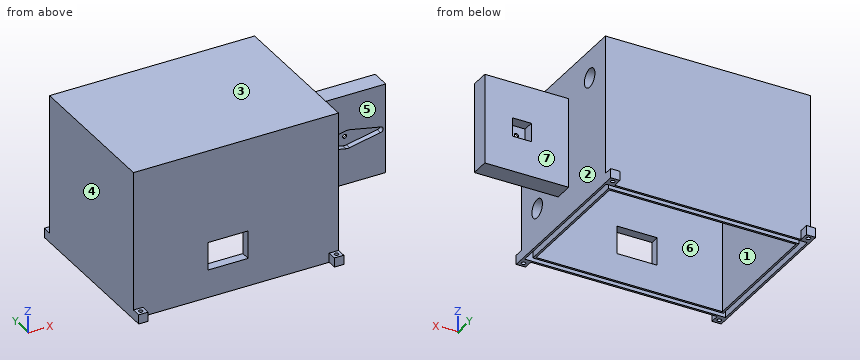
```python
from build123d import *

# Parameters (mm, degrees)
SKETCH_1_W           = 155
SKETCH_1_H           = 80
EXTRUDE_1_DEPTH      = 80
SKETCH_6_W           = 45
SKETCH_6_H           = 80
CUT_EXTRUDE_1_DEPTH  = 35
SKETCH_5_W           = 45
SKETCH_5_H           = 80
CUT_EXTRUDE_2_DEPTH  = 35
SKETCH_7_W           = 100
SKETCH_7_H           = 70
CUT_EXTRUDE_3_DEPTH  = 75
SKETCH_8_W           = 107.8
SKETCH_8_H           = 77.8
SKETCH_8_W_2         = 102.2
SKETCH_8_H_2         = 72.2
CUT_EXTRUDE_4_DEPTH  = 10
SKETCH_9_R           = 5
CUT_EXTRUDE_5_DEPTH  = 10
SKETCH_10_W          = 21.5
SKETCH_10_H          = 15
CUT_EXTRUDE_6_DEPTH  = 10
SKETCH_12_W          = 15.816906699
SKETCH_12_H          = 10
CUT_EXTRUDE_7_DEPTH  = 45
CUT_EXTRUDE_8_DEPTH  = 3
SKETCH_15_W          = 10
SKETCH_15_H          = 10
CUT_EXTRUDE_9_DEPTH  = 6
SKETCH_17_R          = 1.095275866
CUT_EXTRUDE_11_DEPTH = 7
SKETCH_18_W          = 5
SKETCH_18_H          = 5
SKETCH_18_R          = 1.1
EXTRUDE_2_DEPTH      = 5


with BuildPart() as part:
    # 草圖1 → 填料-伸長1 (new body)
    with BuildSketch(Plane.XY):
        with Locations((1.991097826, 5.58988764)):
            Rectangle(SKETCH_1_W, SKETCH_1_H)
    extrude(amount=EXTRUDE_1_DEPTH)

    # 草圖6 → 除料-伸長1 (cut)
    with BuildSketch(Plane(origin=(0, 45.58988764, 0), x_dir=(1, 0, 0), z_dir=(0, 1, 0))):
        with Locations((56.991097826, -40)):
            Rectangle(SKETCH_6_W, SKETCH_6_H)
    extrude(amount=-CUT_EXTRUDE_1_DEPTH, mode=Mode.SUBTRACT)

    # 草圖5 → 除料-伸長2 (cut)
    with BuildSketch(Plane.XZ.offset(34.41011236)):
        with Locations((56.991097826, 40)):
            Rectangle(SKETCH_5_W, SKETCH_5_H)
    extrude(amount=-CUT_EXTRUDE_2_DEPTH, mode=Mode.SUBTRACT)

    # 草圖7 → 除料-伸長3 (cut)
    with BuildSketch(Plane.XY):
        with Locations((-20.508902174, 5.58988764)):
            Rectangle(SKETCH_7_W, SKETCH_7_H)
    extrude(amount=CUT_EXTRUDE_3_DEPTH, mode=Mode.SUBTRACT)

    # 草圖8 → 除料-伸長4 (cut)
    with BuildSketch(Plane(origin=(0, 0, 0), x_dir=(-1, 0, 0), z_dir=(0, 0, -1))):
        with Locations((20.508902174, 5.58988764)):
            Rectangle(SKETCH_8_W, SKETCH_8_H)
        with Locations((20.508902174, 5.58988764)):
            Rectangle(SKETCH_8_W_2, SKETCH_8_H_2, mode=Mode.SUBTRACT)
    extrude(amount=-CUT_EXTRUDE_4_DEPTH, mode=Mode.SUBTRACT)

    # 草圖9 → 除料-伸長5 (cut)
    with BuildSketch(Plane(origin=(34.491097826, 0, 0), x_dir=(0, 0, -1), z_dir=(1, 0, 0))):
        with Locations((-65, 30.58988764)):
            Circle(SKETCH_9_R)
        with Locations((-20, -19.41011236)):
            Circle(SKETCH_9_R)
    extrude(amount=-CUT_EXTRUDE_5_DEPTH, mode=Mode.SUBTRACT)

    # 草圖10 → 除料-伸長6 (cut)
    with BuildSketch(Plane(origin=(0, -34.41011236, 0), x_dir=(-1, 0, 0), z_dir=(0, -1, 0))):
        with Locations((24.758902174, -22.5)):
            Rectangle(SKETCH_10_W, SKETCH_10_H)
    extrude(amount=-CUT_EXTRUDE_6_DEPTH, mode=Mode.SUBTRACT)

    # 草圖12 → 除料-伸長7 (cut)
    with BuildSketch(Plane(origin=(34.491097826, 0, 0), x_dir=(0, 0, -1), z_dir=(1, 0, 0))):
        with Locations((-72.09154665, 5.58988764)):
            Rectangle(SKETCH_12_W, SKETCH_12_H)
        with Locations((-7.90845335, 5.58988764)):
            Rectangle(SKETCH_12_W, SKETCH_12_H)
    extrude(amount=CUT_EXTRUDE_7_DEPTH, mode=Mode.SUBTRACT)

    # 草圖14 → 除料-伸長8 (cut)
    with BuildSketch(Plane(origin=(0, 0.58988764, 0), x_dir=(-1, 0, 0), z_dir=(0, -1, 0))):
        with BuildLine():
            Line((-58.137150435, -35.10282789), (-41.645964254, -38.5))
            ThreePointArc((-41.645964254, -38.5), (-40.145964254, -40), (-41.645964254, -41.5))
            Line((-41.645964254, -41.5), (-58.137150435, -44.89717211))
            ThreePointArc((-58.137150435, -44.89717211), (-59.145964254, -45), (-60.154778073, -44.89717211))
            Line((-60.154778073, -44.89717211), (-76.645964254, -41.5))
            ThreePointArc((-76.645964254, -41.5), (-78.145964254, -40), (-76.645964254, -38.5))
            Line((-76.645964254, -38.5), (-60.154778073, -35.10282789))
            ThreePointArc((-60.154778073, -35.10282789), (-59.145964254, -35), (-58.137150435, -35.10282789))
        make_face()
    extrude(amount=-CUT_EXTRUDE_8_DEPTH, mode=Mode.SUBTRACT)

    # 草圖15 → 除料-伸長9 (cut)
    with BuildSketch(Plane(origin=(0, 10.58988764, 0), x_dir=(1, 0, 0), z_dir=(0, 1, 0))):
        with Locations((59.491097826, -39.816906699)):
            Rectangle(SKETCH_15_W, SKETCH_15_H)
    extrude(amount=-CUT_EXTRUDE_9_DEPTH, mode=Mode.SUBTRACT)

    # 草圖17 → 除料-伸長11 (cut)
    with BuildSketch(Plane(origin=(0, 0.58988764, 0), x_dir=(-1, 0, 0), z_dir=(0, -1, 0))):
        with Locations((-59.145964254, -40)):
            Circle(SKETCH_17_R)
    extrude(amount=-CUT_EXTRUDE_11_DEPTH, mode=Mode.SUBTRACT)

    # 草圖18 → 填料-伸長2 (add)
    with BuildSketch(Plane.XY):
        with Locations((31.991097826, 48.08988764)):
            Rectangle(SKETCH_18_W, SKETCH_18_H)
        with Locations((31.991097826, 48.08988764)):
            Circle(SKETCH_18_R, mode=Mode.SUBTRACT)
        with Locations((-73.008902174, 48.08988764)):
            Rectangle(SKETCH_18_W, SKETCH_18_H)
        with Locations((-73.008902174, 48.08988764)):
            Circle(SKETCH_18_R, mode=Mode.SUBTRACT)
        with Locations((-73.008902174, -36.91011236)):
            Rectangle(SKETCH_18_W, SKETCH_18_H)
        with Locations((-73.008902174, -36.91011236)):
            Circle(SKETCH_18_R, mode=Mode.SUBTRACT)
        with Locations((31.991097826, -36.91011236)):
            Rectangle(SKETCH_18_W, SKETCH_18_H)
        with Locations((31.991097826, -36.91011236)):
            Circle(SKETCH_18_R, mode=Mode.SUBTRACT)
    extrude(amount=EXTRUDE_2_DEPTH)


solid = part.part
```
Model file for the job. Use its own axes, mm. Face numbers are marked on the shaded views. A direction names the side the tool comes from. Give positions to 0.01 mm unless a question says otherwise; leave off trailing zeros. Write each loop counter-clockwise with the first axis right and the second up, starting at its lowest first coordinate (ties: lowest second). Pieces come first, ordered by that corner, then holes. Notation, with made-up numbers: (30, 71) - (63, 71) arc R29 cw to (63, 100) - close; hole circle Ø2 at (-33, 39.25). An arc over 180 degrees is marked (long way). One line per question, with ' | ' between items. Start each with the question number.
(1) Slice it at B-B on z = 73. Write the cut outline in (x, y).
(2) Slice it at C-C on x = 22. Write the cut outline in (y, z).
(3) Slice it at A-A on z = 20. Write the cut outline in (x, y).
(4) Slice it at D-D on y = -2.5. Write the cut outline in (x, z).
(5) 3-axis set-ups, long thin cutter, end or side, ignore diameter. For the marked faces 5, 6 and 7: which of +Z, -Z, +X, -X, +Y, -Y reach the whole face in a straight line?
(6) Pin check, flat tips, straight feed: P1, Ø8, axis at x = 13.5, z = 51.5, coming from the +Y side; P2, Ø11, axis at x = 55.5, z = 40.5, coming from the -Y side; P3, Ø1, axis at x = 21, y = 26, coming from the -Z side; P4, Ø3.5, axis at x = -73.01, y = 48.09, coming from the -Z side. Stop position of each tip, or through.
(7) Wall check: line 1 along X through (y, z) = (-26.5, 4.5); line 2 along X through (y, z) = (-10.5, 69); line 3 along X through (y, z) = (4.2, 40). Give the ranges that are in metal, low to high. Write a range as from..to.
(8) Two-plate mould, pull along X, no slides. Class the marked faces 1, 2, 3 and 4: +X half, -X half, draft (parallel to the pull), parting line (faces both ways), or undercut.
Results below:
1) outline: (-75.51, -34.41) - (34.49, -34.41) - (34.49, 45.59) - (-75.51, 45.59) - close; hole (-70.51, -29.41) - (29.49, -29.41) - (29.49, 40.59) - (-70.51, 40.59) - close
2) outline: (-34.41, 0) - (-33.31, 0) - (-33.31, 10) - (-30.51, 10) - (-30.51, 0) - (-29.41, 0) - (-29.41, 75) - (40.59, 75) - (40.59, 0) - (41.69, 0) - (41.69, 10) - (44.49, 10) - (44.49, 0) - (45.59, 0) - (45.59, 80) - (-34.41, 80) - close
3) outline: (-75.51, -34.41) - (-35.51, -34.41) - (-35.51, -29.41) - (-70.51, -29.41) - (-70.51, 40.59) - (29.49, 40.59) - (29.49, -14.41) - (34.49, -14.41) - (34.49, 0.59) - (79.49, 0.59) - (79.49, 10.59) - (34.49, 10.59) - (34.49, 45.59) - (-75.51, 45.59) - close; (-14.01, -34.41) - (34.49, -34.41) - (34.49, -24.41) - (29.49, -24.41) - (29.49, -29.41) - (-14.01, -29.41) - close
4) outline: (-75.51, 0) - (-74.41, 0) - (-74.41, 10) - (-71.61, 10) - (-71.61, 0) - (-70.51, 0) - (-70.51, 75) - (29.49, 75) - (29.49, 0) - (30.59, 0) - (30.59, 10) - (33.39, 10) - (33.39, 0) - (34.49, 0) - (34.49, 80) - (-75.51, 80) - close
5) face 5: +Z, -Z, +X, -Y | face 6: -Z | face 7: +Z, -Z, +X, +Y
6) P1: y = 45.59 | P2: y = 0.59 | P3: z = 75 | P4: z = 0
7) line 1: -75.51..-74.41, -71.61..-70.51, 29.49..30.59, 33.39..34.49 | line 2: -75.51..-70.51, 29.49..34.49 | line 3: -75.51..-70.51, 29.49..58.05, 60.24..79.49
8) face 1: undercut | face 2: +X half | face 3: draft | face 4: -X half
